```python
from build123d import *

# Parameters (mm, degrees)
F0_W          = 25
F0_H          = 60
F1_DEPTH      = 45
F1_DEPTH_BACK = 45
F3_DEPTH      = 25
F4_W          = 32.849738
F4_H          = 4
F5_DEPTH      = 25
F6_T          = -2.5


with BuildPart() as f1:
    # F0 (on Front) → F1 (new body, two sides)
    with BuildSketch(Plane.XZ) as f1_sk:
        Rectangle(F0_W, F0_H)
    extrude(amount=F1_DEPTH)
    extrude(f1_sk.sketch, amount=-F1_DEPTH_BACK)

    # F2 (on face) → F3 (cut)
    with BuildSketch(Plane(origin=(-12.5, 0, 0), x_dir=(0, -1, 0), z_dir=(-1, 0, 0))):
        Polygon((-45, -30), (12.150262, -30), (-45, -25), align=None)
    extrude(amount=-F3_DEPTH, mode=Mode.SUBTRACT)

    # F4 (on face) → F5 (cut)
    with BuildSketch(Plane(origin=(-12.5, 0, 0), x_dir=(0, -1, 0), z_dir=(-1, 0, 0))):
        with Locations((28.575131, -28)):
            Rectangle(F4_W, F4_H)
    extrude(amount=-F5_DEPTH, mode=Mode.SUBTRACT)

    # F6
    f6_openings = [f1.faces().sort_by_distance(p)[0] for p in [
        (0, -28.575131, -26),
        (0, -12.150262, -28),
        (0, 0, 30),
    ]]
    offset(amount=F6_T, openings=f6_openings)


solid = f1.part
```
Can you work these out from the model? Positions are in its coordinate system, mm. A direction names the side the tool comes from. Coordinates: 2 decimals unless noted, no trailing zeros. Loops run counter-clockwise (first coordinate to the right, second up) from the corner with the lowest first, then second, coordinate; pieces in that order, holes last. Notation, with made-up numbers: (20, 78.5) -> (78, 78.5) arc R30 cw to (78, 113.5) -> close; hole circle Ø3 at (14, -12.5). An arc over 180 degrees is marked (long way). Answer as a JSON object with one key per item and string values.
1) Imagine slicing it at C-C (x = -5). Please give me the cut outline in (y, z), then the cut area to 3 significant figures.
Results:
{"outline": "(-45, -26) -> (-42.5, -26) -> (-42.5, 30) -> (-45, 30) -> close; (-12.15, -30) -> (45, -25) -> (45, 30) -> (42.5, 30) -> (42.5, -22.71) -> (-12.15, -27.49) -> close", "area": "415 mm^2"}
2) If I drill on line 1 (Y direction, x = -8, z = 12); line 2 (X direction, y = 5, z = 11); line 3 (Z direction, x = 10.25, y = -21.5), over which ranges is the centre line in solid material (lowest first)?
Results:
{"line 1": "y = -45 to -42.5, 42.5 to 45", "line 2": "x = -12.5 to -10, 10 to 12.5", "line 3": "z = -26 to 30"}
3) Imagine slicing it at B-B (z = -1). Please give me the cut outline in (x, y).
Results:
{"outline": "(-12.5, -45) -> (12.5, -45) -> (12.5, 45) -> (-12.5, 45) -> close; hole (-10, -42.5) -> (10, -42.5) -> (10, 42.5) -> (-10, 42.5) -> close"}
4) Thinking about a two-plate mould opening in Y: for faces 4 (the face through (0, -42.5, 2)), 5 (the face through (0, -45, 2)), 6 (the face through (-10.2, -3.5, 30)), which applies, pulls with the +Y half, pulls with the -Y half, needs draft (parallel to the pull), parting line crosses it, or undercut?
Results:
{"face 4": "undercut", "face 5": "pulls with the -Y half", "face 6": "needs draft"}
5) For faces 1 (the face through (-10.2, -30.9, -26)), 2 (the face through (12.5, -1, 0)), 3 (the face through (10, -1, 1)), which set-ups out of +Z, -Z, +X, -X, +Y, -Y let a thin tool reach every point of the face, with its end or its side?
Results:
{"face 1": "-Z, +X, -X, -Y", "face 2": "+Z, -Z, +X, +Y, -Y", "face 3": "+Z"}
6) Imagine slicing it at A-A (y = -14.5). Please give me the cut outline in (x, z), then the cut area to 3 significant figures.
Results:
{"outline": "(-12.5, -26) -> (-10, -26) -> (-10, 30) -> (-12.5, 30) -> close; (10, -26) -> (12.5, -26) -> (12.5, 30) -> (10, 30) -> close", "area": "280 mm^2"}
7) Imagine slicing it at D-D (y = 24). Please give me the cut outline in (x, z).
Results:
{"outline": "(-12.5, -26.84) -> (12.5, -26.84) -> (12.5, 30) -> (10, 30) -> (10, -24.33) -> (-10, -24.33) -> (-10, 30) -> (-12.5, 30) -> close"}
8) For P1, Ø8, axis at x = -1, y = 13, coming from the +Z side; P2, Ø8, axis at x = 7, y = -13.5, coming from the -Z side; P3, Ø2, axis at x = 1.5, z = -28.5, coming from the -Y side; P4, Ø1, axis at x = -8, y = 19, coming from the -Z side, each with a flat end and sliding along its axis, tell me the tip position at first contact or that it passes through.
Results:
{"P1": "stops at z = -24.94", "P2": "stops at z = -30", "P3": "stops at y = -12.15", "P4": "stops at z = -27.32"}
